```python
from build123d import *

# Parameters (mm, degrees)
BOSS_EXTRUDE1_DEPTH = 2.921


with BuildPart() as part:
    # Sketch2 → Boss-Extrude1 (new body)
    with BuildSketch(Plane(origin=(0, 0, 0), x_dir=(1, 0, 0), z_dir=(0, 1, 0))):
        Polygon((0, 12.7), (2.921, 12.7), (2.921, 20.447), (5.612336386, 20.447), (5.612336386, 18.25625), (8.390461386, 18.25625), (8.390461386, 20.447), (9.906, 20.447), (9.906, 24.003), (8.390461386, 24.003), (8.390461386, 26.19375), (5.612336386, 26.19375), (5.612336386, 24.003), (2.921, 24.003), (2.921, 31.75), (0, 31.75), (0, 44.45), (15.24, 44.45), (15.24, 24.765), (16.51, 44.45), (19.05, 44.45), (20.32, 24.765), (21.59, 44.45), (24.13, 44.45), (25.4, 24.765), (26.67, 44.45), (29.21, 44.45), (30.48, 24.765), (31.75, 44.45), (34.29, 44.45), (35.56, 24.765), (36.83, 44.45), (39.37, 44.45), (40.64, 24.765), (41.91, 44.45), (44.45, 44.45), (45.72, 24.765), (46.99, 44.45), (49.53, 44.45), (50.8, 24.765), (50.8, 19.685), (49.53, 0), (46.99, 0), (45.72, 19.685), (44.45, 0), (41.91, 0), (40.64, 19.685), (39.37, 0), (36.83, 0), (35.56, 19.685), (34.29, 0), (31.75, 0), (30.48, 19.685), (29.21, 0), (26.67, 0), (25.4, 19.685), (24.13, 0), (21.59, 0), (20.32, 19.685), (19.05, 0), (16.51, 0), (15.24, 19.685), (15.24, 0), (0, 0), align=None)
        with BuildLine():
            Line((48.025626044, 40.817203674), (46.99, 24.765))
            Line((46.99, 24.765), (46.99, 19.685))
            Line((46.99, 19.685), (48.025626044, 3.632796326))
            ThreePointArc((48.025626044, 3.632796326), (48.26, 3.398422369), (48.494373956, 3.632796326))
            Line((48.494373956, 3.632796326), (49.53, 19.685))
            Line((49.53, 19.685), (49.53, 24.765))
            Line((49.53, 24.765), (48.494373956, 40.817203674))
            ThreePointArc((48.494373956, 40.817203674), (48.26, 41.051577631), (48.025626044, 40.817203674))
        make_face(mode=Mode.SUBTRACT)
        with BuildLine():
            Line((42.945626044, 40.817203674), (41.91, 24.765))
            Line((41.91, 24.765), (41.91, 19.685))
            Line((41.91, 19.685), (42.945626044, 3.632796326))
            ThreePointArc((42.945626044, 3.632796326), (43.18, 3.398422369), (43.414373956, 3.632796326))
            Line((43.414373956, 3.632796326), (44.45, 19.685))
            Line((44.45, 19.685), (44.45, 24.765))
            Line((44.45, 24.765), (43.414373956, 40.817203674))
            ThreePointArc((43.414373956, 40.817203674), (43.18, 41.051577631), (42.945626044, 40.817203674))
        make_face(mode=Mode.SUBTRACT)
        with BuildLine():
            Line((37.865626044, 40.817203674), (36.83, 24.765))
            Line((36.83, 24.765), (36.83, 19.685))
            Line((36.83, 19.685), (37.865626044, 3.632796326))
            ThreePointArc((37.865626044, 3.632796326), (38.1, 3.398422369), (38.334373956, 3.632796326))
            Line((38.334373956, 3.632796326), (39.37, 19.685))
            Line((39.37, 19.685), (39.37, 24.765))
            Line((39.37, 24.765), (38.334373956, 40.817203674))
            ThreePointArc((38.334373956, 40.817203674), (38.1, 41.051577631), (37.865626044, 40.817203674))
        make_face(mode=Mode.SUBTRACT)
        with BuildLine():
            Line((32.785626044, 40.817203674), (31.75, 24.765))
            Line((31.75, 24.765), (31.75, 19.685))
            Line((31.75, 19.685), (32.785626044, 3.632796326))
            ThreePointArc((32.785626044, 3.632796326), (33.02, 3.398422369), (33.254373956, 3.632796326))
            Line((33.254373956, 3.632796326), (34.29, 19.685))
            Line((34.29, 19.685), (34.29, 24.765))
            Line((34.29, 24.765), (33.254373956, 40.817203674))
            ThreePointArc((33.254373956, 40.817203674), (33.02, 41.051577631), (32.785626044, 40.817203674))
        make_face(mode=Mode.SUBTRACT)
        with BuildLine():
            Line((27.705626044, 40.817203674), (26.67, 24.765))
            Line((26.67, 24.765), (26.67, 19.685))
            Line((26.67, 19.685), (27.705626044, 3.632796326))
            ThreePointArc((27.705626044, 3.632796326), (27.94, 3.398422369), (28.174373956, 3.632796326))
            Line((28.174373956, 3.632796326), (29.21, 19.685))
            Line((29.21, 19.685), (29.21, 24.765))
            Line((29.21, 24.765), (28.174373956, 40.817203674))
            ThreePointArc((28.174373956, 40.817203674), (27.94, 41.051577631), (27.705626044, 40.817203674))
        make_face(mode=Mode.SUBTRACT)
        with BuildLine():
            Line((22.625626044, 40.817203674), (21.59, 24.765))
            Line((21.59, 24.765), (21.59, 19.685))
            Line((21.59, 19.685), (22.625626044, 3.632796326))
            ThreePointArc((22.625626044, 3.632796326), (22.86, 3.398422369), (23.094373956, 3.632796326))
            Line((23.094373956, 3.632796326), (24.13, 19.685))
            Line((24.13, 19.685), (24.13, 24.765))
            Line((24.13, 24.765), (23.094373956, 40.817203674))
            ThreePointArc((23.094373956, 40.817203674), (22.86, 41.051577631), (22.625626044, 40.817203674))
        make_face(mode=Mode.SUBTRACT)
        with BuildLine():
            Line((17.545626044, 40.817203674), (16.51, 24.765))
            Line((16.51, 24.765), (16.51, 19.685))
            Line((16.51, 19.685), (17.545626044, 3.632796326))
            ThreePointArc((17.545626044, 3.632796326), (17.78, 3.398422369), (18.014373956, 3.632796326))
            Line((18.014373956, 3.632796326), (19.05, 19.685))
            Line((19.05, 19.685), (19.05, 24.765))
            Line((19.05, 24.765), (18.014373956, 40.817203674))
            ThreePointArc((18.014373956, 40.817203674), (17.78, 41.051577631), (17.545626044, 40.817203674))
        make_face(mode=Mode.SUBTRACT)
    extrude(amount=BOSS_EXTRUDE1_DEPTH)


solid = part.part
```
Verification items for the finished model (mm, model axes). A direction names the side the tool comes from. Give positions to 0.01 mm unless a question says otherwise; leave off trailing zeros.
1. Mould release check, pull along X, two halves, no side actions. Record for faces 1 (the flat face through (48, 1, -44.45)), 2 (the flat face through (15.24, 1, -10)): released by +X, released by -X, zero draft, split by the parting line, or undercut.
2. Set-up check for faces 3 (the flat face through (31.75, 1, -22)), 4 (the flat face through (48, 1, 0)): record each of +Z, -Z, +X, -X, +Y, -Y from which the full face is reachable in a straight line by a thin tool's end or side.
3. Section check A-A, the plane z = -22.5. Count the separate pieces of the cut face and the enclosed holes in it, then the cut area to 3 significant figures.
4. Thickness scan on line 1 (Z direction, x = 3, y = 2.8); line 2 (Z direction, x = 2.5, y = 0.5). Record the ranges inside material, lowest first.
5. Go/stop test with flat-tipped pins: pin 1 Ø1 at (x, z) = (45, -28.5) entering from -Y; pin 2 Ø1 at (y, z) = (0.5, -39) entering from +X; pin 3 Ø0.9 at (y, z) = (1, -16.5) entering from -X; pin 4 Ø1.5 at (y, z) = (1, -22) entering from -X. Record where each tip stops, or that it passes through.
Geometry says:
1. face 1: zero draft
1. face 2: undercut
2. face 3: +Y, -Y
2. face 4: +Z, +X, -X, +Y, -Y
3. separate pieces: 8
3. enclosed holes: 0
3. area: 67.5 mm2
4. line 1: z = -44.45 to -24, -20.45 to 0
4. line 2: z = -44.45 to -31.75, -12.7 to 0
5. pin 1: stops at y = 0
5. pin 2: stops at x = 49.91
5. pin 3: stops at x = 2.92
5. pin 4: stops at x = 9.91
